Autodesk Inventor part; units mm, degrees
ref_plane "Work Plane1" through (0, 0, -2.8) normal (0, 0, -1) x (-1, 0, 0)
ref_plane "YZ Plane" through (0, 0, 0) normal (1, 0, 0) x (0, 1, 0)
ref_plane "XZ Plane" through (0, 0, 0) normal (0, 1, 0) x (-1, 0, 0)
sketch "Sketch1" plane through (0, 0, 0) normal (0, 0, 1) x (1, 0, 0)
  circle A0 centre (0, 0) radius 4
  dimension "d0" = 8
extrude "Extrusion1" add sketch "Sketch1" along normal mid plane 8
sketch "Sketch2" plane through (0, 0, 4) normal (0, 0, 1) x (1, 0, 0)
  circle A0 centre (0, 0) radius 2.4
  line L0 (-2.2627, 0.8) -> (-0.8, 0.8)
  line L1 (-0.8, 0.8) -> (-0.8, 2.2627)
  line L2 (0.8, 2.2627) -> (0.8, 0.8)
  line L3 (0.8, 0.8) -> (2.2627, 0.8)
  line L4 (2.2627, -0.8) -> (0.8, -0.8)
  line L5 (0.8, -0.8) -> (0.8, -2.2627)
  line L6 (-0.8, -2.2627) -> (-0.8, -0.8)
  line L7 (-0.8, -0.8) -> (-2.2627, -0.8)
  dimension "d3" = 4.8
  dimension "d4" = 1.6
extrude "Extrusion2" cut sketch "Sketch2" against normal through all contours A0 L4 L5 L6 L7 L0 L1 L2 L3
ref_plane "Work Plane1" through (0, 0, -2.8) normal (0, 0, -1) x (-1, 0, 0)
sketch "Sketch3" plane through (0, 0, -2.8) normal (0, 0, -1) x (-1, 0, 0)
  circle A0 centre (0, 0) radius 4
  circle A1 centre (0, 0) radius 4
  circle A2 centre (0, 0) radius 3
  dimension "d8" = 6
extrude "Extrusion3" cut sketch "Sketch3" against normal blind 5.6
sketch "Sketch4" plane through (0, 0, -4) normal (0, 0, -1) x (-1, 0, 0)
  circle A0 centre (4, -4) radius 2.5
  point P0 (0, 0)
  dimension "d11" = 4
  dimension "d12" = 4
  dimension "d13" = 5
extrude "Extrusion4" cut sketch "Sketch4" against normal up to surface (1.2 mm away)
pattern_circular "Circular Pattern1" count 4 over 360 about axis through (0, 0, -10) along (0, 0, 1) of "Extrusion4"
sketch "Sketch5" plane through (0, 0, 0) normal (0, 1, 0) x (-1, 0, 0)
  line L0 (-0.8, 4) -> (-0.8, -4)
  line L1 (0.8, 4) -> (0.8, -4)
  line L2 (4, 2.8) -> (-4, 2.8)
  line L3 (-1.518, -2.8) -> (1.518, -2.8)
  line L4 (-0.8, -2.8) -> (0.8, -2.8)
  line L5 (0.8, -2.8) -> (0.8, 2.8)
  line L6 (0.8, 2.8) -> (-0.8, 2.8)
  line L7 (-0.8, 2.8) -> (-0.8, -2.8)
  point P0 (0, 0)
extrude "Extrusion5" cut sketch "Sketch5" along normal through all both and the other way through all
fillet "Fillet1" radius 0.3 16 edges at (-0.8, 0.8, 0) (-0.8, -0.8, 0) (0.8, -0.8, 0) (0.8, 0.8, 0) (-2.2627, -0.8, 0) (-2.2627, 0.8, 0) (-0.8, 2.2627, 3.4) (0.8, 2.2627, 3.4) (2.2627, 0.8, 0) (2.2627, -0.8, 0) (0.8, -2.2627, 3.4) (-0.8, -2.2627, 3.4) (0.8, 2.2627, -3.4) (-0.8, 2.2627, -3.4) (0.8, -2.2627, -3.4) (-0.8, -2.2627, -3.4)
properties part number "3713" material "Steel"
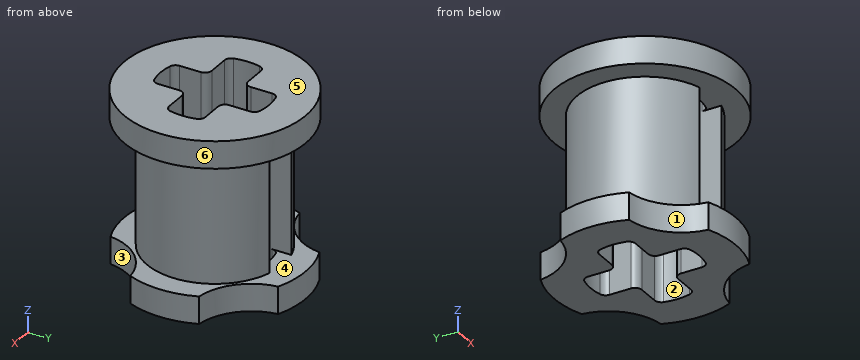
For this review, take the finished solid that the model builds, in its own axes (mm). Face numbers are marked on the shaded views. A direction names the side the tool comes from. Round coordinates to 2 decimals unless told otherwise and drop trailing zeros. Order: outer loops, then holes, each group sorted by start corner. A loop starts at its lowest first (then second) coordinate and runs counter-clockwise, first axis right, second up. Notation, with made-up numbers: M -37.75,57 L 18.25,57 A23 ccw 18.25,88 Z; hole C -28.75,70.25 d1. An arc over 180 degrees is marked long. Write each question's results on one line, items separated by ' | '. Start each with the question number.
1. To check wall thickness, follow L1, parallel to X at y = 0, z = 1.5; L2, parallel to Z at x = 3.25, y = -1; L3, parallel to Z at x = 1.75, y = -3.5. State the ranges of each line that lie inside material, in increasing order. Write a range as [from, to].
2. Add section D-D (x = 0). State the section outline as (y, z) points.
3. Tool access review of the marked faces 1, 2 and 3: name each direction out of +Z, -Z, +X, -X, +Y, -Y from which nothing blocks a thin tool from reaching the whole face with its end or side.
4. Draft analysis for pull direction Z (two halves, no side actions). For the marked faces 4, 5 and 6, state which applies: pulls with the +Z half, pulls with the -Z half, needs draft (parallel to the pull), parting line crosses it, or undercut.
5. Add section A-A (z = 0.75). State the section outline as (x, y) points, then the cut area to 3 significant figures.
6. Clearance check with flat-ended pins moving along their axes: pin 1 Ø2 at (y, z) = (2, 1.5) entering from +X; pin 2 Ø2.5 at (x, y) = (-1.5, -0.5) entering from +Z; pin 3 Ø0.5 at (x, z) = (1.5, -1) entering from +Y; pin 4 Ø1 at (x, z) = (-1.5, 1.5) entering from -Y. State where each tip first meets the part, or that it passes through.
7. Add section C-C (y = 0). State the section outline as (x, z) points.
8. Add section B-B (z = 3). State the section outline as (x, y) points, then the cut area to 3 significant figures.
Output values:
1) L1: [-3, -2.4], [2.4, 3] | L2: [-4, -2.8], [2.8, 4] | L3: [2.8, 4]
2) outline: M -4,-4 L -2.4,-4 L -2.4,-2.8 L -4,-2.8 Z; M -4,2.8 L -2.4,2.8 L -2.4,4 L -4,4 Z; M 2.4,-4 L 4,-4 L 4,-2.8 L 2.4,-2.8 Z; M 2.4,2.8 L 4,2.8 L 4,4 L 2.4,4 Z
3) face 1: -Z, -X, -Y | face 2: +Z, -Z | face 3: -Z, +X, -Y
4) face 4: undercut | face 5: pulls with the +Z half | face 6: needs draft
5) outline: M -2.33,-0.57 A2.4 cw -2.33,0.57 A0.3 cw -2.04,0.8 L -1.1,0.8 A0.3 ccw -0.8,1.1 L -0.8,2.89 A3 ccw -0.8,-2.89 L -0.8,-1.1 A0.3 ccw -1.1,-0.8 L -2.04,-0.8 A0.3 cw Z; M 0.8,-2.89 A3 ccw 0.8,2.89 L 0.8,1.1 A0.3 ccw 1.1,0.8 L 2.04,0.8 A0.3 cw 2.33,0.57 A2.4 cw 2.33,-0.57 A0.3 cw 2.04,-0.8 L 1.1,-0.8 A0.3 ccw 0.8,-1.1 Z | area: 13.8 mm^2
6) pin 1: x = 2.83 | pin 2: z = 4 | pin 3: y = 2.73 | pin 4: y = -2.83
7) outline: M -4,-4 L -2.4,-4 L -2.4,4 L -4,4 L -4,2.8 L -3,2.8 L -3,-2.8 L -4,-2.8 Z; M 2.4,-4 L 4,-4 L 4,-2.8 L 3,-2.8 L 3,2.8 L 4,2.8 L 4,4 L 2.4,4 Z
8) outline: C 0,0 d8; hole M -2.33,-0.57 A0.3 ccw -2.04,-0.8 L -1.1,-0.8 A0.3 cw -0.8,-1.1 L -0.8,-2.04 A0.3 ccw -0.57,-2.33 A2.4 ccw 0.57,-2.33 A0.3 ccw 0.8,-2.04 L 0.8,-1.1 A0.3 cw 1.1,-0.8 L 2.04,-0.8 A0.3 ccw 2.33,-0.57 A2.4 ccw 2.33,0.57 A0.3 ccw 2.04,0.8 L 1.1,0.8 A0.3 cw 0.8,1.1 L 0.8,2.04 A0.3 ccw 0.57,2.33 A2.4 ccw -0.57,2.33 A0.3 ccw -0.8,2.04 L -0.8,1.1 A0.3 cw -1.1,0.8 L -2.04,0.8 A0.3 ccw -2.33,0.57 A2.4 ccw Z | area: 37.8 mm^2
